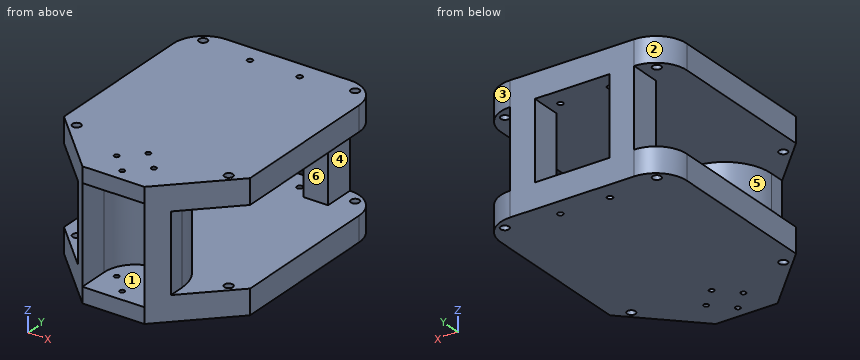
```python
from build123d import *

# Parameters (mm, degrees)
SKETCH1_R           = 0.883567379
SKETCH1_R_2         = 0.896609669
SKETCH1_R_3         = 0.8
SKETCH1_R_4         = 1.35
BOSS_EXTRUDE1_DEPTH = 8
SKETCH2_W           = 8
SKETCH2_H           = 10
BOSS_EXTRUDE3_DEPTH = 25
BOSS_EXTRUDE4_START = 33
SKETCH1_2_R         = 0.883567379
SKETCH1_2_R_2       = 0.896609669
SKETCH1_2_R_3       = 0.8
SKETCH1_2_R_4       = 1.35
BOSS_EXTRUDE4_DEPTH = 8
CUT_EXTRUDE1_DEPTH  = 3
CUT_EXTRUDE2_START  = 28
CUT_EXTRUDE2_DEPTH  = 3
BOSS_EXTRUDE5_DEPTH = 25
CUT_EXTRUDE3_DEPTH  = 41
FILLET5_R           = 10


with BuildPart() as part:
    # Sketch1 → Boss-Extrude1 (new body)
    with BuildSketch(Plane.XY):
        Polygon((-30, 20.206387144), (0, 20.206387144), (30, 20.206387144), (30, -59.793612856), (-30, -59.793612856), align=None)
        with Locations((-8, 14.206387144)):
            Circle(SKETCH1_R, mode=Mode.SUBTRACT)
        with Locations((8, 14.206387144)):
            Circle(SKETCH1_R_2, mode=Mode.SUBTRACT)
        with Locations((0, -43.793612856)):
            Circle(SKETCH1_R_3, mode=Mode.SUBTRACT)
        with Locations((6, -49.793612856)):
            Circle(SKETCH1_R_3, mode=Mode.SUBTRACT)
        with Locations((0, -55.793612856)):
            Circle(SKETCH1_R_3, mode=Mode.SUBTRACT)
        with Locations((-6, -49.793612856)):
            Circle(SKETCH1_R_3, mode=Mode.SUBTRACT)
        with Locations((-24.5, 16.206387144)):
            Circle(SKETCH1_R_4, mode=Mode.SUBTRACT)
        with Locations((24.5, 16.206387144)):
            Circle(SKETCH1_R_4, mode=Mode.SUBTRACT)
        with Locations((-24.5, -41.793612856)):
            Circle(SKETCH1_R_4, mode=Mode.SUBTRACT)
        with Locations((24.5, -41.793612856)):
            Circle(SKETCH1_R_4, mode=Mode.SUBTRACT)
    extrude(amount=BOSS_EXTRUDE1_DEPTH)

    # Sketch2 → Boss-Extrude3 (add)
    with BuildSketch(Plane.XY.offset(8)):
        with Locations((-16, 15.206387144)):
            Rectangle(SKETCH2_W, SKETCH2_H)
        with Locations((16, 15.206387144)):
            Rectangle(SKETCH2_W, SKETCH2_H)
    extrude(amount=BOSS_EXTRUDE3_DEPTH)

    # Sketch1<2> → Boss-Extrude4 (add)
    with BuildSketch(Plane.XY.offset(BOSS_EXTRUDE4_START)):
        Polygon((-30, 20.206387144), (0, 20.206387144), (30, 20.206387144), (30, -59.793612856), (-30, -59.793612856), align=None)
        with Locations((-8, 14.206387144)):
            Circle(SKETCH1_2_R, mode=Mode.SUBTRACT)
        with Locations((8, 14.206387144)):
            Circle(SKETCH1_2_R_2, mode=Mode.SUBTRACT)
        with Locations((0, -43.793612856)):
            Circle(SKETCH1_2_R_3, mode=Mode.SUBTRACT)
        with Locations((6, -49.793612856)):
            Circle(SKETCH1_2_R_3, mode=Mode.SUBTRACT)
        with Locations((0, -55.793612856)):
            Circle(SKETCH1_2_R_3, mode=Mode.SUBTRACT)
        with Locations((-6, -49.793612856)):
            Circle(SKETCH1_2_R_3, mode=Mode.SUBTRACT)
        with Locations((-24.5, 16.206387144)):
            Circle(SKETCH1_2_R_4, mode=Mode.SUBTRACT)
        with Locations((24.5, 16.206387144)):
            Circle(SKETCH1_2_R_4, mode=Mode.SUBTRACT)
        with Locations((-24.5, -41.793612856)):
            Circle(SKETCH1_2_R_4, mode=Mode.SUBTRACT)
        with Locations((24.5, -41.793612856)):
            Circle(SKETCH1_2_R_4, mode=Mode.SUBTRACT)
    extrude(amount=BOSS_EXTRUDE4_DEPTH)

    # Sketch3 → Cut-Extrude1 (cut)
    with BuildSketch(Plane.XY.offset(8)):
        with BuildLine():
            Line((-10, -49.793612856), (-10, -59.793612856))
            Line((-10, -59.793612856), (10, -59.793612856))
            Line((10, -59.793612856), (10, -49.793612856))
            ThreePointArc((10, -49.793612856), (0, -39.793612856), (-10, -49.793612856))
        make_face()
    extrude(amount=-CUT_EXTRUDE1_DEPTH, mode=Mode.SUBTRACT)

    # Sketch3<2> → Cut-Extrude2 (cut)
    with BuildSketch(Plane.XY.offset(8).offset(CUT_EXTRUDE2_START)):
        with BuildLine():
            Line((-10, -49.793612856), (-10, -59.793612856))
            Line((-10, -59.793612856), (10, -59.793612856))
            Line((10, -59.793612856), (10, -49.793612856))
            ThreePointArc((10, -49.793612856), (0, -39.793612856), (-10, -49.793612856))
        make_face()
    extrude(amount=-CUT_EXTRUDE2_DEPTH, mode=Mode.SUBTRACT)

    # Sketch5 → Boss-Extrude5 (add)
    with BuildSketch(Plane(origin=(0, 0, 33), x_dir=(-1, 0, 0), z_dir=(0, 0, -1))):
        with BuildLine():
            Line((-15, -49.793612856), (-15, -59.793612856))
            Line((-15, -59.793612856), (-10, -59.793612856))
            Line((-10, -59.793612856), (-10, -49.793612856))
            ThreePointArc((-10, -49.793612856), (0, -39.793612856), (10, -49.793612856))
            Line((10, -49.793612856), (10, -59.793612856))
            Line((10, -59.793612856), (15, -59.793612856))
            Line((15, -59.793612856), (15, -49.793612856))
            ThreePointArc((15, -49.793612856), (0, -34.793612856), (-15, -49.793612856))
        make_face()
    extrude(amount=BOSS_EXTRUDE5_DEPTH)

    # Sketch7 → Cut-Extrude3 (cut)
    with BuildSketch(Plane.XY.offset(41)):
        Polygon((30, -39.793612856), (30, -59.793612856), (10, -59.793612856), align=None)
        Polygon((-30, -39.793612856), (-30, -59.793612856), (-10, -59.793612856), align=None)
    extrude(amount=-CUT_EXTRUDE3_DEPTH, mode=Mode.SUBTRACT)

    # Fillet5
    fillet5_edges = [part.edges().sort_by_distance(p)[0] for p in [
        (-30, 20.206387144, 37),
        (-30, 20.206387144, 4),
        (30, 20.206387144, 4),
        (30, 20.206387144, 37),
    ]]
    fillet(fillet5_edges, radius=FILLET5_R)


solid = part.part
```
Model file for the job. Use its own axes, mm. Face numbers are marked on the shaded views. A direction names the side the tool comes from. Give positions to 0.01 mm unless a question says otherwise; leave off trailing zeros. Loops run counter-clockwise (first coordinate to the right, second up) from the corner with the lowest first, then second, coordinate; pieces in that order, holes last. Notation, with made-up numbers: (88, 51.5) - (117, 51.5) arc R7 ccw to (117, 57.5) - close; hole circle Ø10 at (33, 53.5). An arc over 180 degrees is marked (long way). One line per item, written item: value. Start each with the question number.
1. Pull direction X, two halves, no side cores. Call the marked faces 1, 2 and 3: pulls with the +X half, pulls with the -X half, needs draft (parallel to the pull), parting line crosses it, or undercut.
2. Probe L1, parallel to Y at x = 0, z = 38.5; L2, parallel to Z at x = -20.5, y = -34.5; L3, parallel to Y at x = 24.5, z = 34.75. List the from-to ranges inside material, lowest first. Write a range as from..to.
3. Slice it at A-A (y = -5.5). List the corners of the cut face in (x, z).
4. Pin check, flat tips, straight feed: pin 1 (11 mm diameter, centred on y = 15.5, z = 17, fed in from +X); pin 2 (3 mm diameter, centred on y = 13.5, z = 16.5, fed in from -X); pin 3 (1 mm diameter, centred on x = 17, z = 8, fed in from -Y). Stop position of each tip, or through.
5. Slice it at C-C (x = -8). List the corners of the cut face in (y, z), plus the area to 3 significant figures.
6. Slice it at D-D (y = -46.5). List the corners of the cut face in (x, z).
7. Which spindle directions (+Z, -Z, +X, -X, +Y, -Y) get a long thin tool onto all of the face, cutting with end or side? Do the marked faces 4, 5 and 6. Say none if no direction does.
8. Slice it at B-B (z = 14). List the corners of the cut face in (x, y), plus the area to 3 significant figures.
Solution:
1. face 1: undercut
1. face 2: pulls with the -X half
1. face 3: pulls with the +X half
2. L1: y = -59.79..-56.59, -54.99..-44.59, -42.99..20.21
2. L2: z = 0..8, 33..41
2. L3: y = -45.29..-43.14, -40.44..14.86, 17.56..19.14
3. outline: (-30, 0) - (30, 0) - (30, 8) - (-30, 8) - close; (-30, 33) - (30, 33) - (30, 41) - (-30, 41) - close
4. pin 1: stops at x = 20
4. pin 2: stops at x = -20
4. pin 3: stops at y = -53.29
5. outline: (-59.79, 0) - (13.32, 0) - (13.32, 8) - (-37.11, 8) - (-37.11, 33) - (13.32, 33) - (13.32, 41) - (-59.79, 41) - (-59.79, 36) - (-43.79, 36) - (-43.79, 5) - (-59.79, 5) - close; (15.09, 0) - (20.21, 0) - (20.21, 8) - (15.09, 8) - close; (15.09, 33) - (20.21, 33) - (20.21, 41) - (15.09, 41) - close
5. area: 1,320 mm^2
6. outline: (-23.29, 0) - (23.29, 0) - (23.29, 8) - (14.63, 8) - (14.63, 33) - (23.29, 33) - (23.29, 41) - (-23.29, 41) - (-23.29, 33) - (-14.63, 33) - (-14.63, 8) - (-23.29, 8) - close; hole (-9.44, 5) - (9.44, 5) - (9.44, 36) - (-9.44, 36) - close
7. face 4: +X, +Y, -Y
7. face 5: none
7. face 6: +X, -X
8. outline: (-20, 10.21) - (-12, 10.21) - (-12, 20.21) - (-20, 20.21) - close; (-15, -54.79) - (-10, -59.79) - (-10, -49.79) arc R10 cw to (10, -49.79) - (10, -59.79) - (15, -54.79) - (15, -49.79) arc R15 ccw to (-15, -49.79) - close; (12, 10.21) - (20, 10.21) - (20, 20.21) - (12, 20.21) - close
8. area: 431 mm^2
